The listing builds one solid part. Answer for the finished solid, in the listing's coordinates (mm). Face numbers are marked on the shaded views. A direction names the side the tool comes from. Coordinates: 2 decimals unless noted, no trailing zeros. Order: outer loops, then holes, each group sorted by start corner. A loop starts at its lowest first (then second) coordinate and runs counter-clockwise, first axis right, second up. Notation, with made-up numbers: (29, 81) - (77, 81) arc R27 ccw to (77, 120) - close; hole circle Ø7 at (75.25, 76.25). An arc over 180 degrees is marked (long way). Use a Markdown table: item, result. Add a question column.
Item 1: The part is cut by section A-A, the plane z = 0. State how many separate pieces and enclosed holes the cut face has, then the cut area to 3 significant figures.
Item 2: The part is cut by section C-C, the plane x = 22. Give the vertices of the cut face in (y, z), then the cut area to 3 significant figures.
Item 3: The mould has two halves that part along Z. Classify the marked faces 4, 5 and 6: released by +Z, released by -Z, zero draft, split by the parting line, or undercut.
Item 4: Find the intervals of material crossed by line 1 along Y through (x, z) = (26.65, 0); line 2 along Y through (x, z) = (1, 6); line 3 along X through (y, z) = (1, 7.5), in increasing order.
Item 5: For the marked faces 1, 2 and 3, determine the directions among +Z, -Z, +X, -X, +Y, -Y from which every point of the face is accessible in a straight line to the end or side of a thin tool.
Item 6: Flat-ended cylindrical pins translate along their axes: P1, Ø2, axis at x = 3, z = 2, coming from the +Y side; P2, Ø4, axis at y = -8.13, z = -8.13, coming from the +X side; P3, Ø8, axis at y = 0, z = -11.5, coming from the +X side. Find the tip coordinate at first contact, or state that the pin passes through.
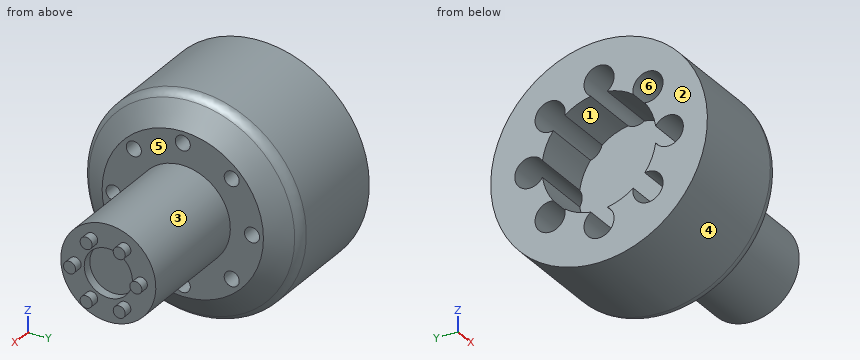
from build123d import *

# Parameters (mm, degrees)
SKETCH2_R           = 1.25
CUT_EXTRUDE1_DEPTH  = 21.98
SKETCH3_R           = 2.5
CUT_EXTRUDE2_DEPTH  = 15.98
SKETCH4_R           = 9.5
CUT_EXTRUDE3_DEPTH  = 10
FILLET2_R           = 2
SKETCH6_R           = 4
CUT_EXTRUDE5_DEPTH  = 1.5
SKETCH7_R           = 1
BOSS_EXTRUDE1_DEPTH = 1.5


with BuildPart() as part:
    # Sketch1 → Revolve1 (revolve)
    with BuildSketch(Plane(origin=(0, 0, 0), x_dir=(1, 0, 0), z_dir=(0, 1, 0))):
        Polygon((7.143835403, 7.9), (7.143835403, 13.4), (4.13367975, 18), (-13.836164597, 18), (-13.836164597, 0), (7.143835403, 0), (27.143835403, 0), (27.143835403, 7.9), align=None)
    revolve(axis=Axis((-26.115988439, 0, 0), (1, 0, 0)))

    # Sketch2 → Cut-Extrude1 (cut, through all)
    with BuildSketch(Plane(origin=(7.143835403, 0, 0), x_dir=(0, 0, -1), z_dir=(1, 0, 0))):
        with Locations((0, 11.5)):
            Circle(SKETCH2_R)
        with Locations((8.131727984, 8.131727984)):
            Circle(SKETCH2_R)
        with Locations((11.5, 0)):
            Circle(SKETCH2_R)
        with Locations((8.131727984, -8.131727984)):
            Circle(SKETCH2_R)
        with Locations((0, -11.5)):
            Circle(SKETCH2_R)
        with Locations((-8.131727984, -8.131727984)):
            Circle(SKETCH2_R)
        with Locations((-11.5, 0)):
            Circle(SKETCH2_R)
        with Locations((-8.131727984, 8.131727984)):
            Circle(SKETCH2_R)
    extrude(amount=-CUT_EXTRUDE1_DEPTH, mode=Mode.SUBTRACT)

    # Sketch3 → Cut-Extrude2 (cut)
    with BuildSketch(Plane.ZY.offset(13.836164597)):
        with Locations((0, 11.5)):
            Circle(SKETCH3_R)
        with Locations((8.131727984, 8.131727984)):
            Circle(SKETCH3_R)
        with Locations((11.5, 0)):
            Circle(SKETCH3_R)
        with Locations((8.131727984, -8.131727984)):
            Circle(SKETCH3_R)
        with Locations((0, -11.5)):
            Circle(SKETCH3_R)
        with Locations((-8.131727984, -8.131727984)):
            Circle(SKETCH3_R)
        with Locations((-11.5, 0)):
            Circle(SKETCH3_R)
        with Locations((-8.131727984, 8.131727984)):
            Circle(SKETCH3_R)
    extrude(amount=-CUT_EXTRUDE2_DEPTH, mode=Mode.SUBTRACT)

    # Sketch4 → Cut-Extrude3 (cut)
    with BuildSketch(Plane.ZY.offset(13.836164597)):
        Circle(SKETCH4_R)
    extrude(amount=-CUT_EXTRUDE3_DEPTH, mode=Mode.SUBTRACT)

    # Fillet2
    fillet2_edges = [part.edges().sort_by_distance(p)[0] for p in [
        (4.13367975, 0, 18),
    ]]
    fillet(fillet2_edges, radius=FILLET2_R)

    # Sketch6 → Cut-Extrude5 (cut)
    with BuildSketch(Plane(origin=(27.143835403, 0, 0), x_dir=(0, 0, -1), z_dir=(1, 0, 0))):
        Circle(SKETCH6_R)
    extrude(amount=-CUT_EXTRUDE5_DEPTH, mode=Mode.SUBTRACT)

    # Sketch7 → Boss-Extrude1 (add)
    with BuildSketch(Plane(origin=(27.143835403, 0, 0), x_dir=(0, 0, -1), z_dir=(1, 0, 0))):
        with Locations((0, 5.5)):
            Circle(SKETCH7_R)
        with Locations((4.763139721, 2.75)):
            Circle(SKETCH7_R)
        with Locations((4.763139721, -2.75)):
            Circle(SKETCH7_R)
        with Locations((0, -5.5)):
            Circle(SKETCH7_R)
        with Locations((-4.763139721, -2.75)):
            Circle(SKETCH7_R)
        with Locations((-4.763139721, 2.75)):
            Circle(SKETCH7_R)
    extrude(amount=BOSS_EXTRUDE1_DEPTH)


solid = part.part
Solution:
| question | item | result |
|---|---|---|
| 1 | separate pieces | 3 |
| 1 | enclosed holes | 0 |
| 1 | area | 686 mm2 |
| 2 | outline | circle Ø15.8 at (0, 0) |
| 2 | area | 196 mm2 |
| 3 | face 4 | split by the parting line |
| 3 | face 5 | zero draft |
| 3 | face 6 | undercut |
| 4 | line 1 | y = -7.9 to -4, 4 to 7.9 |
| 4 | line 2 | y = -16.97 to -9.44, -6.83 to 6.83, 9.44 to 16.97 |
| 4 | line 3 | x = -3.84 to 27.14 |
| 5 | face 1 | -X |
| 5 | face 2 | +Z, -Z, -X, +Y, -Y |
| 5 | face 3 | +X |
| 6 | P1 | stops at y = 17.97 |
| 6 | P2 | stops at x = 7.14 |
| 6 | P3 | stops at x = 27.14 |
